from build123d import *

# Parameters (mm, degrees)
F0_R     = 25.4
F1_DEPTH = 2.54
F2_R     = 25.4
F2_R_2   = 22.987
F3_DEPTH = 16.51
F6_W     = 10.16
F6_H     = 2.54
F8_W     = 10.16
F8_H     = 2.54
F10_R    = 1.27
F11_R    = 0.508


with BuildPart() as f1:
    # F0 (on Top) → F1 (new body)
    with BuildSketch(Plane.XY):
        Circle(F0_R)
    extrude(amount=F1_DEPTH)

    # F2 (on face) → F3 (join)
    with BuildSketch(Plane.XY.offset(2.54)):
        Circle(F2_R)
        Circle(F2_R_2, mode=Mode.SUBTRACT)
    extrude(amount=F3_DEPTH)

    # F6 (on offset) → F7 (join, up to the next surface of F1)
    with BuildSketch(Plane.XZ.offset(16.51)):
        with Locations((0, 13.97)):
            Rectangle(F6_W, F6_H)
    extrude(until=Until.NEXT)

    # F8 (on offset) → F9 (join, up to the next surface of F1)
    with BuildSketch(Plane.XZ.offset(-16.51)):
        with Locations((0, 5.08)):
            Rectangle(F8_W, F8_H)
    extrude(until=Until.NEXT, dir=(0, 1, 0))

    # F10
    f10_edges = [f1.edges().sort_by_distance(p)[0] for p in [
        (-25.4, 0, 0),
    ]]
    fillet(f10_edges, radius=F10_R)

    # F11
    f11_edges = [f1.edges().sort_by_distance(p)[0] for p in [
        (0, -16.51, 15.24),
        (-5.08, -19.464324, 15.24),
        (0, -22.987, 15.24),
        (5.08, -19.464324, 15.24),
        (-5.08, -16.51, 13.97),
        (-5.08, -19.464324, 12.7),
        (-5.08, -22.418648, 13.97),
        (5.08, -16.51, 13.97),
        (5.08, -22.418648, 13.97),
        (5.08, -19.464324, 12.7),
        (0, -16.51, 12.7),
        (25.028026, 0, 0.371974),
        (-25.4, 0, 1.27),
        (-24.13, 0, 0),
        (0, 16.51, 6.35),
        (-5.08, 19.464324, 6.35),
        (0, 22.987, 6.35),
        (5.08, 19.464324, 6.35),
        (5.08, 16.51, 5.08),
        (-5.08, 16.51, 5.08),
        (0, 16.51, 3.81),
        (5.08, 22.418648, 5.08),
        (5.08, 19.464324, 3.81),
        (-5.08, 19.464324, 3.81),
        (-5.08, 22.418648, 5.08),
        (0, -22.987, 12.7),
        (0, 22.987, 3.81),
    ]]
    fillet(f11_edges, radius=F11_R)


solid = f1.part
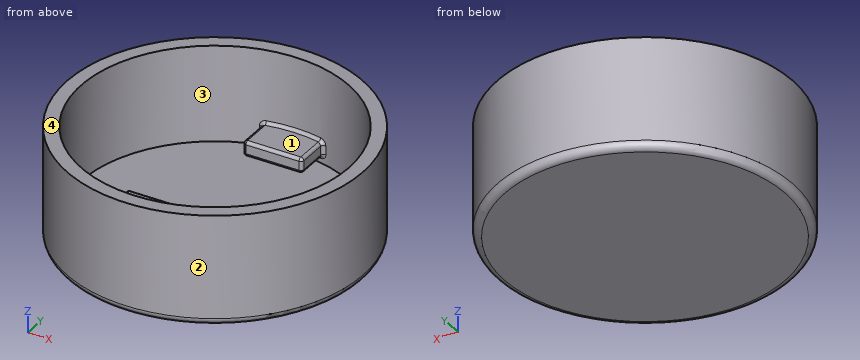
CAD build for the part. Positions are in the model's coordinates, mm. Face numbers are marked on the shaded views. Give positions to 0.01 mm unless a question says otherwise; leave off trailing zeros. Loops run counter-clockwise (first coordinate to the right, second up) from the corner with the lowest first, then second, coordinate; pieces in that order, holes last. Notation, with made-up numbers: M 20,67 L 25,67 A35 cw 25,101 Z; hole C 80,22.25 d11. An arc over 180 degrees is marked long. Answer in a Markdown table with one row per item. Add a question column.
Item 1: Probe probe 1 along Y at (x, z) = (0, 13.75); probe 2 along Y at (x, z) = (0, 7.25); probe 3 along Z at (x, y) = (21, -3). List the from-to ranges inside material, lowest first.
Item 2: Band-saw the part on C-C on z = 9.5. Give the cut face in (x, y), then the cut area to 3 significant figures.
Item 3: Drop flat-ended pins along their axis: P1, Ø3, axis at y = -4, z = 10.5, coming from the +X side; P2, Ø3, axis at y = -10.5, z = 9, coming from the +X side; P3, Ø23, axis at x = 8, y = -4, coming from the +Z side. Give the stop position or say it passes through.
Item 4: Band-saw the part on A-A on x = 0. Give the cut face in (y, z).
Item 5: Band-saw the part on B-B on y = 0. Give the cut face in (x, z).
Item 6: Mould opens along Y. For the marked faces 1, 2, 3 and 4 say: +Y half, -Y half, draft (parallel to the pull), parting line (faces both ways), or undercut.
Reply:
| question | item | result |
|---|---|---|
| 1 | probe 1 | y = -25.4 to -16.51, 22.99 to 25.4 |
| 1 | probe 2 | y = -25.4 to -22.99, 22.99 to 25.4 |
| 1 | probe 3 | z = 0 to 2.54 |
| 2 | outline | C 0,0 d50.8; hole C 0,0 d45.97 |
| 2 | area | 367 mm^2 |
| 3 | P1 | stops at x = 25.28 |
| 3 | P2 | stops at x = 23.75 |
| 3 | P3 | stops at z = 2.54 |
| 4 | outline | M -25.4,1.27 A1.27 ccw -24.13,0 L 24.13,0 A1.27 ccw 25.4,1.27 L 25.4,19.05 L 22.99,19.05 L 22.99,6.86 A0.51 cw 22.48,6.35 L 17.02,6.35 A0.51 ccw 16.51,5.84 L 16.51,4.32 A0.51 ccw 17.02,3.81 L 22.48,3.81 A0.51 cw 22.99,3.3 L 22.99,2.54 L -22.99,2.54 L -22.99,12.19 A0.51 cw -22.48,12.7 L -17.02,12.7 A0.51 ccw -16.51,13.21 L -16.51,14.73 A0.51 ccw -17.02,15.24 L -22.48,15.24 A0.51 cw -22.99,15.75 L -22.99,19.05 L -25.4,19.05 Z |
| 5 | outline | M -25.4,1.27 A1.27 ccw -24.13,0 L 24.13,0 A1.27 ccw 25.4,1.27 L 25.4,19.05 L 22.99,19.05 L 22.99,2.54 L -22.99,2.54 L -22.99,19.05 L -25.4,19.05 Z |
| 6 | face 1 | undercut |
| 6 | face 2 | parting line |
| 6 | face 3 | undercut |
| 6 | face 4 | draft |
